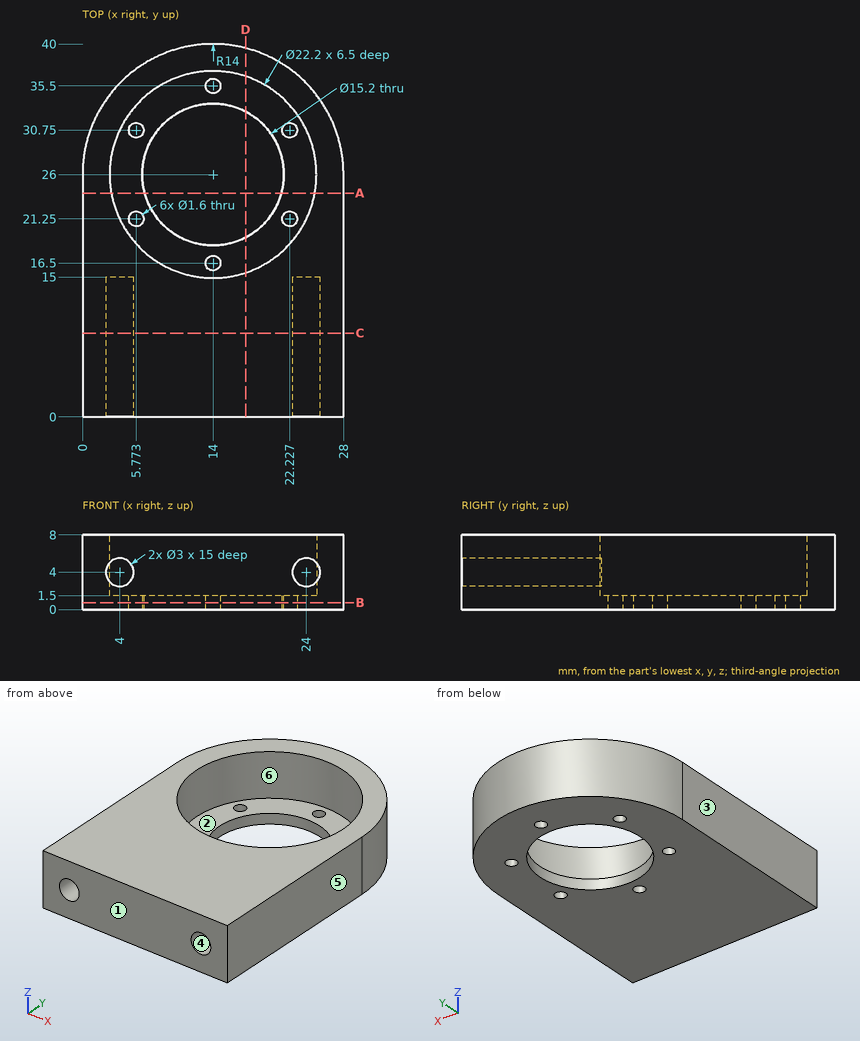
Check sheet for the drawn part. Datum: minimum x, y, z corner. Units: mm. A direction names the side the tool comes from. Coordinates: 2 decimals unless noted, no trailing zeros. Order: outer loops, then holes, each group sorted by start corner. A loop starts at its lowest first (then second) coordinate and runs counter-clockwise, first axis right, second up. Notation, with made-up numbers: (-10, 2.25) -> (17, 2.25) arc R30 cw to (17, 32.25) -> close; hole circle Ø5 at (-13, 46.5). An arc over 180 degrees is marked (long way). Write each question's results on one line, items separated by ' | '. Start each with the question number.
1) Section check D-D (x = 17.5). Enter the section's corners in (y, z) (1 decimal), and give its area (3 significant figures).
2) Draft check along Y on the marked faces 1, 2 and 3. Enter one of: pulls with the +Y half, pulls with the -Y half, needs draft (parallel to the pull), parting line crosses it, or undercut.
3) Material ranges on line 1 along Y through (x, z) = (14, 0.75); line 2 along Y through (x, z) = (14, 6.25); line 3 along X through (y, z) = (30.5, 0.75) (1 decimal), recorded low to high.
4) Set-up check for the marked faces 4, 5 and 6: record each of +Z, -Z, +X, -X, +Y, -Y from which the full face is reachable in a straight line by a thin tool's end or side.
5) Section check C-C (y = 9). Enter the section's corners in (x, z), and give its area (3 significant figures).
6) Section check A-A (y = 24). Enter the section's corners in (x, z).
7) Section check B-B (z = 0.75). Enter the section's corners in (x, y).
8) Depth check by flat-ended pin: pin 1 (1 mm diameter, centred on x = 17.5, z = 7, fed in from +Y) (1 decimal); pin 2 (2 mm diameter, centred on x = 5.77, y = 30.75, fed in from +Z); pin 3 (1.8 mm diameter, centred on x = 24, z = 4, fed in from +Y). Enter the tip coordinate at first touch or a pass-through.
Checked values:
1) outline: (0, 0) -> (19.3, 0) -> (19.3, 1.5) -> (15.5, 1.5) -> (15.5, 8) -> (0, 8) -> close; (32.7, 0) -> (39.6, 0) -> (39.6, 8) -> (36.5, 8) -> (36.5, 1.5) -> (32.7, 1.5) -> close | area: 159 mm²
2) face 1: pulls with the -Y half | face 2: undercut | face 3: needs draft
3) line 1: 0 to 15.7, 17.3 to 18.4, 33.6 to 34.7, 36.3 to 40 | line 2: 0 to 14.9, 37.1 to 40 | line 3: 0.7 to 5, 6.5 to 7.9, 20.1 to 21.5, 23 to 27.3
4) face 4: -Y | face 5: +Z, -Z, +X, +Y, -Y | face 6: +Z
5) outline: (0, 0) -> (28, 0) -> (28, 8) -> (0, 8) -> close; hole circle Ø3 at (4, 4); hole circle Ø3 at (24, 4) | area: 210 mm²
6) outline: (0, 0) -> (6.67, 0) -> (6.67, 1.5) -> (3.08, 1.5) -> (3.08, 8) -> (0, 8) -> close; (21.33, 0) -> (28, 0) -> (28, 8) -> (24.92, 8) -> (24.92, 1.5) -> (21.33, 1.5) -> close
7) outline: (0, 0) -> (28, 0) -> (28, 26) arc R14 ccw to (0, 26) -> close; hole circle Ø1.6 at (5.77, 21.25); hole circle Ø1.6 at (5.77, 30.75); hole circle Ø15.2 at (14, 26); hole circle Ø1.6 at (14, 16.5); hole circle Ø1.6 at (14, 35.5); hole circle Ø1.6 at (22.23, 21.25); hole circle Ø1.6 at (22.23, 30.75)
8) pin 1: y = 39.7 | pin 2: z = 1.5 | pin 3: y = 36.64
